For this review, take the finished solid that the model builds, in its own axes (mm). Round coordinates to 2 decimals unless told otherwise and drop trailing zeros. Loops run counter-clockwise (first coordinate to the right, second up) from the corner with the lowest first, then second, coordinate; pieces in that order, holes last. Notation, with made-up numbers: (-27, -36.75) -> (-7, -36.75) arc R12 cw to (-7, -14.75) -> close; hole circle Ø1 at (-0.5, 18.5). An arc over 180 degrees is marked (long way). One line per question, with ' | ' between items. Start each with the question number.
1. Wall thickness on line 1 along X through (y, z) = (3.05, 0); line 2 along X through (y, z) = (4.4, 0.5); line 3 along X through (y, z) = (2.95, -8.75): over which ranges is each line inside the solid? List them lowest first.
2. Consider section A-A (z = 0). Write out the cut boundary in (x, y), and give its area (3 significant figures).
3. Consider section B-B (y = 3.4). Write out the cut boundary in (x, z).
```python
from build123d import *

# Parameters (mm, degrees)
BOSS_EXTRUDE1_DEPTH = 5
CUT_EXTRUDE1_REACH  = 63.033
SKETCH2_R           = 1.5


with BuildPart() as part:
    # Sketch1 → Boss-Extrude1 (new body)
    with BuildSketch(Plane(origin=(0, 0, 0), x_dir=(1, 0, 0), z_dir=(0, 1, 0))):
        with BuildLine():
            Line((-50, 10), (50, 10))
            ThreePointArc((50, 10), (60, 0), (50, -10))
            Line((50, -10), (-50, -10))
            ThreePointArc((-50, -10), (-60, 0), (-50, 10))
        make_face()
    extrude(amount=BOSS_EXTRUDE1_DEPTH)

    # Sketch2 → Cut-Extrude1 (cut, up to next)
    with BuildSketch(Plane(origin=(0, 5, 0), x_dir=(1, 0, 0), z_dir=(0, 1, 0)), mode=Mode.PRIVATE) as cut_extrude1_sk1:
        with Locations(Location((-50, 0, 0), (0, 0, 270))):
            Circle(SKETCH2_R)
    cut_extrude1_tool1 = extrude(cut_extrude1_sk1.sketch, amount=-CUT_EXTRUDE1_REACH, mode=Mode.PRIVATE) & part.part
    # Sketch2 → Cut-Extrude1 (cut, up to next)
    with BuildSketch(Plane(origin=(0, 5, 0), x_dir=(1, 0, 0), z_dir=(0, 1, 0)), mode=Mode.PRIVATE) as cut_extrude1_sk2:
        with Locations(Location((50, 0, 0), (0, 0, 270))):
            Circle(SKETCH2_R)
    cut_extrude1_tool2 = extrude(cut_extrude1_sk2.sketch, amount=-CUT_EXTRUDE1_REACH, mode=Mode.PRIVATE) & part.part
    add(cut_extrude1_tool1.solids().sort_by_distance((-50, 5, 0))[0], mode=Mode.SUBTRACT)
    add(cut_extrude1_tool2.solids().sort_by_distance((50, 5, 0))[0], mode=Mode.SUBTRACT)


solid = part.part
```
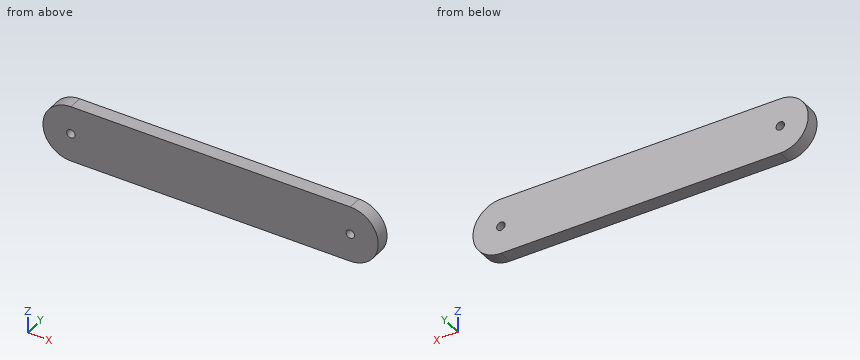
Answer block:
1) line 1: x = -60 to -51.5, -48.5 to 48.5, 51.5 to 60 | line 2: x = -59.99 to -51.41, -48.59 to 48.59, 51.41 to 59.99 | line 3: x = -54.84 to 54.84
2) outline: (-60, 0) -> (-51.5, 0) -> (-51.5, 5) -> (-60, 5) -> close; (-48.5, 0) -> (48.5, 0) -> (48.5, 5) -> (-48.5, 5) -> close; (51.5, 0) -> (60, 0) -> (60, 5) -> (51.5, 5) -> close | area: 570 mm2
3) outline: (-50, -10) -> (50, -10) arc R10 ccw to (50, 10) -> (-50, 10) arc R10 ccw to start; hole circle Ø3 at (-50, 0); hole circle Ø3 at (50, 0)
